Input: part model. Units: mm. Frame: model coordinates. Coordinates: 2 decimals unless noted, no trailing zeros. Write each loop counter-clockwise with the first axis right and the second up, starting at its lowest first coordinate (ties: lowest second). Pieces come first, ordered by that corner, then holes. Notation, with made-up numbers: (38, -33.75) -> (66, -33.75) arc R15 cw to (66, -17.75) -> close; hole circle Ø3 at (-9, -25). An arc over 180 degrees is marked (long way). Use one line per item in the form item = value. Start each with the question number.
(1) First-contact query: pin 1 (12 mm diameter, centred on x = -10.5, y = -23, fed in from +Z); pin 2 (8 mm diameter, centred on y = -15, z = 8, fed in from -X); pin 3 (3 mm diameter, centred on x = -17.5, y = -31, fed in from +Z). Flat tips, straight axial feed; report the tip coordinate or a pass-through.
(2) Cut plane B-B on z = 0. Return the cut outline in (x, y), plus the area to 3 significant figures.
(3) Ray query, line 1 along X through (y, z) = (-7, 14); line 2 along X through (y, z) = (-14, 13); line 3 along Z through (x, y) = (2, -16). Return the intervals inside material, ascending.
(4) Cut plane A-A on x = 0. Return the cut outline in (y, z).
(5) Cut plane C-C on y = -14.5. Return the cut outline in (x, z).
```python
from build123d import *

# Parameters (mm, degrees)
F0_R     = 23.761832
F1_DEPTH = 38.1
F2_SIZE  = 5.08
F3_SIZE  = 5.08


with BuildPart() as f1:
    # F0 (on Front) → F1 (new body)
    with BuildSketch(Plane.XZ):
        Circle(F0_R)
    extrude(amount=F1_DEPTH)

    # F2
    f2_edges = [f1.edges().sort_by_distance(p)[0] for p in [
        (-23.761832, -38.1, 0),
    ]]
    chamfer(f2_edges, length=F2_SIZE)

    # F3
    f3_edges = [f1.edges().sort_by_distance(p)[0] for p in [
        (-23.761832, 0, 0),
    ]]
    chamfer(f3_edges, length=F3_SIZE)


solid = f1.part
```
Values:
q1.pin_1 = 23.33
q1.pin_2 = -23.42
q1.pin_3 = 17.57
q2.outline = (-23.76, -33.02) -> (-18.68, -38.1) -> (18.68, -38.1) -> (23.76, -33.02) -> (23.76, -5.08) -> (18.68, 0) -> (-18.68, 0) -> (-23.76, -5.08) -> close
q2.area = 1,760 mm2
q3.line_1 = -19.2 to 19.2
q3.line_2 = -19.89 to 19.89
q3.line_3 = -23.68 to 23.68
q4.outline = (-38.1, -18.68) -> (-33.02, -23.76) -> (-5.08, -23.76) -> (0, -18.68) -> (0, 18.68) -> (-5.08, 23.76) -> (-33.02, 23.76) -> (-38.1, 18.68) -> close
q5.outline = circle Ø47.52 at (0, 0)
